```python
from build123d import *

# Parameters (mm, degrees)
SKETCH1_W           = 88
SKETCH1_H           = 71.8
BOSS_EXTRUDE1_DEPTH = 30
SKETCH2_W           = 20
SKETCH2_H           = 15
SKETCH2_W_2         = 16
SKETCH2_W_3         = 18
BOSS_EXTRUDE2_DEPTH = 5


with BuildPart() as part:
    # Sketch1 → Boss-Extrude1 (new body)
    with BuildSketch(Plane(origin=(0, 0, 0), x_dir=(1, 0, 0), z_dir=(0, 1, 0))):
        Rectangle(SKETCH1_W, SKETCH1_H)
    extrude(amount=BOSS_EXTRUDE1_DEPTH)

    # Sketch2 → Boss-Extrude2 (add)
    with BuildSketch(Plane.XY.offset(35.9)):
        with Locations((-24, 15)):
            Rectangle(SKETCH2_W, SKETCH2_H)
        with Locations((-2, 15)):
            Rectangle(SKETCH2_W_2, SKETCH2_H)
        with Locations((22, 15)):
            Rectangle(SKETCH2_W_3, SKETCH2_H)
    extrude(amount=BOSS_EXTRUDE2_DEPTH)


solid = part.part
```
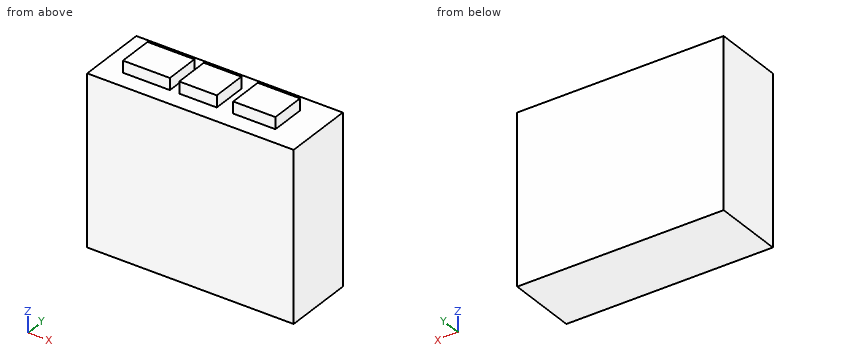
Work out the finished part from the listing and answer in its coordinate system (mm). Round coordinates to 2 decimals unless told otherwise and drop trailing zeros. Write each loop counter-clockwise with the first axis right and the second up, starting at its lowest first coordinate (ties: lowest second). Pieces come first, ordered by that corner, then holes.
1) A cutting plane is placed at B-B on x = -28.5. Determine the outline of the cut face in (y, z), and give its area (3 significant figures).
2) Flat-ended cylindrical pins translate along their axes: P1, Ø5.5, axis at x = -1, z = 39, coming from the -Y side; P2, Ø1.5, axis at x = 21.5, z = 39, coming from the +Y side; P3, Ø1.5, axis at y = 15.5, z = 38, coming from the +X side. Find the tip coordinate at first contact, or state that the pin passes through.
3) A cutting plane is placed at A-A on y = 15.75. Determine the outline of the cut face in (x, z).
4) Consider probe 1 along Z at (x, y) = (-39.5, 28). Determine where the line is inside the solid, lowest interval first.
5) A cutting plane is placed at C-C on y = 4.25. Determine the outline of the cut face in (x, z), and give its area (3 significant figures).
Entries:
1. outline: (0, -35.9) - (30, -35.9) - (30, 35.9) - (22.5, 35.9) - (22.5, 40.9) - (7.5, 40.9) - (7.5, 35.9) - (0, 35.9) - close
1. area: 2,230 mm2
2. P1: stops at y = 7.5
2. P2: stops at y = 22.5
2. P3: stops at x = 31
3. outline: (-44, -35.9) - (44, -35.9) - (44, 35.9) - (31, 35.9) - (31, 40.9) - (13, 40.9) - (13, 35.9) - (6, 35.9) - (6, 40.9) - (-10, 40.9) - (-10, 35.9) - (-14, 35.9) - (-14, 40.9) - (-34, 40.9) - (-34, 35.9) - (-44, 35.9) - close
4. probe 1: z = -35.9 to 35.9
5. outline: (-44, -35.9) - (44, -35.9) - (44, 35.9) - (-44, 35.9) - close
5. area: 6,320 mm2
